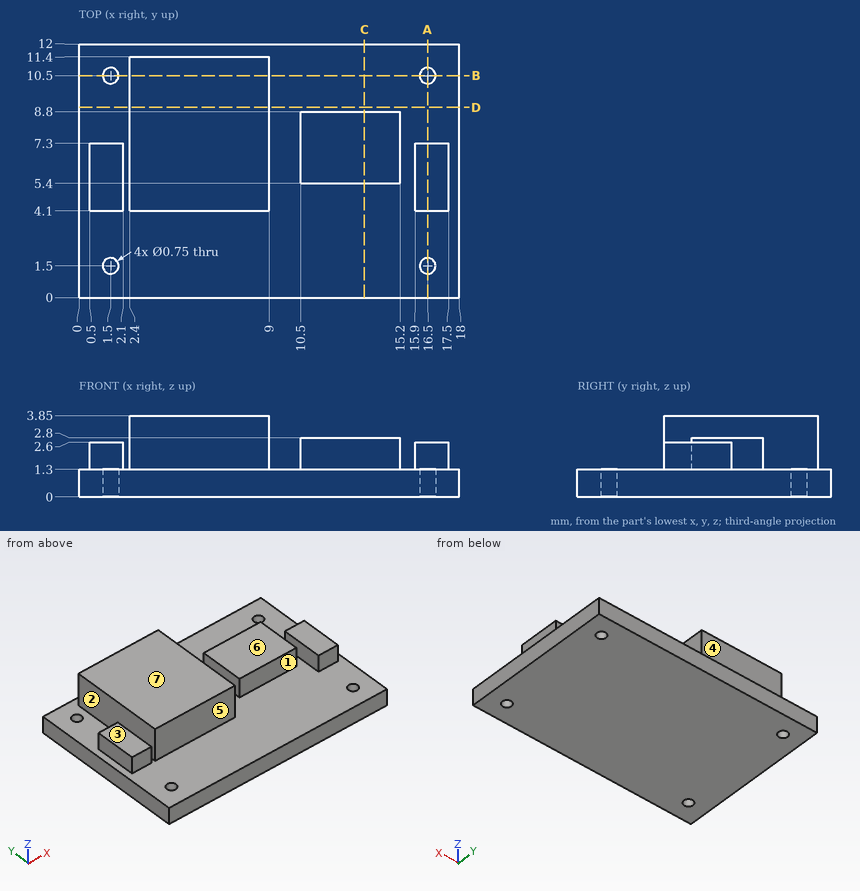
Source: three-view drawing plus pictorial views. Frame: mm from the lowest corner of the part. A direction names the side the tool comes from. Round coordinates to 2 decimals unless told otherwise and drop trailing zeros. Loops run counter-clockwise (first coordinate to the right, second up) from the corner with the lowest first, then second, coordinate; pieces in that order, holes last. Notation, with made-up numbers: M 75,82 L 88,82 A34 cw 88,112 Z; hole C 28,58.5 d5. An arc over 180 degrees is marked long. Put each result on its own line as item: value. Start each with the question number.
(1) Contact query for flat-ended pins moving along their axis: pin 1 Ø1 at (x, z) = (17, 2) entering from +Y; pin 2 Ø0.6 at (y, z) = (5.5, 2) entering from +X; pin 3 Ø1.6 at (x, z) = (14, 2) entering from -Y; pin 4 Ø0.6 at (y, z) = (5, 2) entering from -X. Output: stop coordinate, or through.
(2) Draft query along X for the marked faces 1, 2 and 3. Return one class per face: +X half, -X half, draft (parallel to the pull), parting line (faces both ways), or undercut.
(3) Section query B-B (y = 10.5). Return loops of the section in (x, z) (3 decimals).
(4) Set-up query: the marked faces 4, 5, 6 and 7. Return all of +Z, -Z, +X, -X, +Y, -Y with unobstructed straight access to the full face (end or side cutting, diameter ignored); none if empty.
(5) Section query A-A (x = 16.5). Return loops of the section in (y, z) (3 decimals).
(6) Section query D-D (y = 9). Return loops of the section in (x, z).
(7) Section query C-C (x = 13.5). Return loops of the section in (y, z), then the cut area to 3 significant figures.
(8) Material intervals for line 1 along Y through (x, z) = (1.5, 1.05) (3 decimals); line 2 along X through (y, z) = (4.25, 3); line 3 along Z through (x, y) = (2, 4.5), sorted ascending. Write a range as [from, to].
Findings below:
1. pin 1: stops at y = 7.3
1. pin 2: stops at x = 17.5
1. pin 3: stops at y = 0
1. pin 4: stops at x = 0.5
2. face 1: undercut
2. face 2: undercut
2. face 3: draft
3. outline: M 0,0 L 1.125,0 L 1.125,1.3 L 0,1.3 Z; M 1.875,0 L 16.125,0 L 16.125,1.3 L 9,1.3 L 9,3.85 L 2.4,3.85 L 2.4,1.3 L 1.875,1.3 Z; M 16.875,0 L 18,0 L 18,1.3 L 16.875,1.3 Z
4. face 4: +Z, +X, -X, +Y
4. face 5: +Z, +X, -X, -Y
4. face 6: +Z, +X, +Y, -Y
4. face 7: +Z, +X, -X, +Y, -Y
5. outline: M 0,0 L 1.125,0 L 1.125,1.3 L 0,1.3 Z; M 1.875,0 L 10.125,0 L 10.125,1.3 L 7.3,1.3 L 7.3,2.6 L 4.1,2.6 L 4.1,1.3 L 1.875,1.3 Z; M 10.875,0 L 12,0 L 12,1.3 L 10.875,1.3 Z
6. outline: M 0,0 L 18,0 L 18,1.3 L 9,1.3 L 9,3.85 L 2.4,3.85 L 2.4,1.3 L 0,1.3 Z
7. outline: M 0,0 L 12,0 L 12,1.3 L 8.8,1.3 L 8.8,2.8 L 5.4,2.8 L 5.4,1.3 L 0,1.3 Z
7. area: 20.7 mm2
8. line 1: y = [0, 1.125], [1.875, 10.125], [10.875, 12]
8. line 2: x = [2.4, 9]
8. line 3: z = [0, 2.6]
